Check sheet for the drawn part. Datum: minimum x, y, z corner. Units: mm. Give positions to 0.01 mm unless a question says otherwise; leave off trailing zeros. Order: outer loops, then holes, each group sorted by start corner. A loop starts at its lowest first (then second) coordinate and runs counter-clockwise, first axis right, second up. Notation, with made-up numbers: (12, 35.5) - (38, 35.5) arc R12 ccw to (38, 50.5) - close; hole circle Ø1 at (77.5, 88). An arc over 180 degrees is marked (long way). Answer as a JSON object with one key per item and string values. Group by question number.
(1) Section check A-A (x = 15.5). Record the boundary of the cut face in (y, z).
(2) Mould release check, pull along Y, two halves, no side actions. Record for the marked faces 1 and 2: +Y half, -Y half, draft (parallel to the pull), parting line (faces both ways), or undercut.
(3) Depth check by flat-ended pin: pin 1 Ø4 at (y, z) = (8.5, 6) entering from -X; pin 2 Ø2 at (x, y) = (17.5, 15) entering from +Z (1 decimal); pin 3 Ø3 at (x, z) = (3, 7) entering from +Y; pin 4 Ø3 at (x, z) = (17.5, 2.5) entering from +Y. Enter the tip coordinate at first touch or a pass-through.
(4) Thickness scan on line 1 (Z direction, x = 19, y = 9.7); line 2 (Y direction, x = 11, z = 9.7); line 3 (Z direction, x = 21.25, y = 10.5). Record the ranges inside material, lowest first.
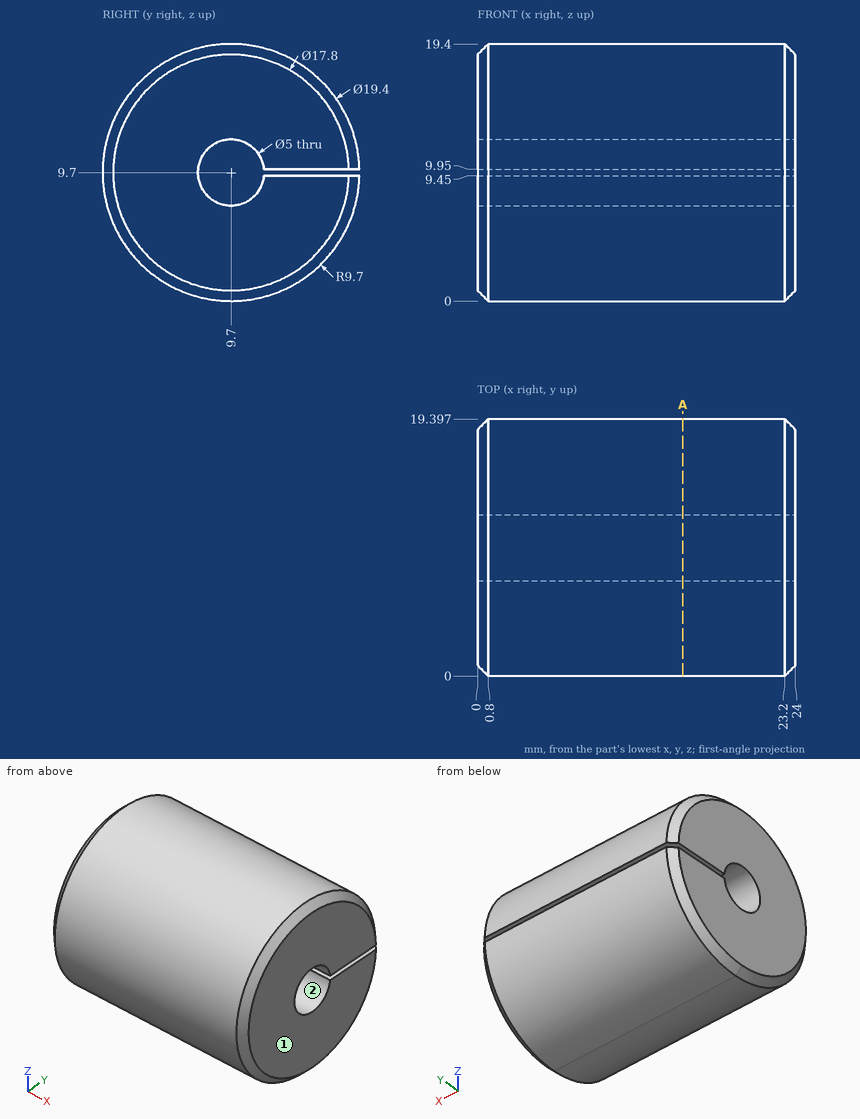
Solutions:
{
 "1": {"outline": "(12.19, 9.45) arc R2.5 cw (long way) to (12.19, 9.95) - (19.4, 9.95) arc R9.7 ccw (long way) to (19.4, 9.45) - close"},
 "2": {"face 1": "draft", "face 2": "undercut"},
 "3": {"pin 1": "stops at x = 0", "pin 2": "stops at z = 18.4", "pin 3": "stops at y = 19.33", "pin 4": "stops at y = 17.55"},
 "4": {"line 1": "z = 0 to 7.2, 12.2 to 19.4", "line 2": "y = 0 to 7.2", "line 3": "z = 0.03 to 7.33, 12.07 to 19.37"}
}
